Design review of the part built by this model. Coordinates are the model's own, in mm. Face numbers are marked on the shaded views. A direction names the side the tool comes from. Round coordinates to 2 decimals unless told otherwise and drop trailing zeros. Write each loop counter-clockwise with the first axis right and the second up, starting at its lowest first coordinate (ties: lowest second). Pieces come first, ordered by that corner, then holes. Notation, with made-up numbers: (68.5, 11) -> (112.5, 11) arc R26 ccw to (112.5, 34) -> close; hole circle Ø9 at (52, 65). An arc over 180 degrees is marked (long way). One line per question, with ' | ' between items. Start each with the question number.
1) Insertion check: pin 1 Ø3 at (y, z) = (0.5, -5) entering from +X; pin 2 Ø2 at (y, z) = (-1.5, -4.5) entering from +X. Each pin has a flat end and moves straight along its axis. Give the tip position at first contact, or say it passes through.
2) Consider section C-C (z = -3.75). Give the boundary of the cut face in (x, y).
3) For probe 1 along Y at (x, z) = (0, -2.35); probe 2 along X at (y, z) = (0.35, -1.5); probe 3 along X at (y, z) = (0.9, -3.1), list the stretches that pass through material, from the lowest coordinate up.
4) Consider section D-D (z = -0.8). Give the boundary of the cut face in (x, y), then the cut area to 3 significant figures.
5) For the marked faces 1 and 2, list the 3-axis set-ups (+Z, -Z, +X, -X, +Y, -Y) from which the entire face can be reached by the end or side of a thin tool; tool diameter is ignored.
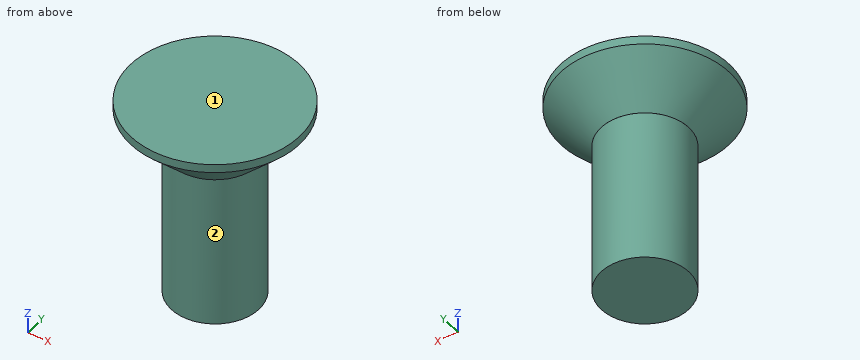
Autodesk Inventor part; units mm, degrees
ref_plane "YZ Plane" through (0, 0, 0) normal (1, 0, 0) x (0, 1, 0)
ref_plane "XZ Plane" through (0, 0, 0) normal (0, 1, 0) x (-1, 0, 0)
ref_plane "XY Plane" through (0, 0, 0) normal (0, 0, 1) x (1, 0, 0)
sketch "スケッチ1" plane through (0, 0, 0) normal (0, 0, 1) x (1, 0, 0)
  circle A0 centre (0, 0) radius 1.3
  dimension "d0" = 2.6
extrude "押し出し1" add sketch "スケッチ1" against normal blind 6
sketch "スケッチ2" plane through (0, 0, 0) normal (0, 0, 1) x (1, 0, 0)
  circle A0 centre (0, 0) radius 2.5
  dimension "d3" = 5
extrude "押し出し2" add sketch "スケッチ2" against normal blind 1.45
chamfer "面取り3" distance 1.2 angle 45 1 edges at (-2.5, 0, -1.45)
thread "ねじ1"
properties part number "ネジ皿m2.6,06" material "鋼、高強度、低合金"
From the geometry:
1) pin 1: stops at x = 1.3 | pin 2: stops at x = 1.2
2) outline: circle Ø2.6 at (0, 0)
3) probe 1: y = -1.3 to 1.3 | probe 2: x = -1.25 to 1.25 | probe 3: x = -0.94 to 0.94
4) outline: circle Ø3.9 at (0, 0) | area: 12.0 mm2
5) face 1: +Z, +X, -X, +Y, -Y | face 2: -Z
